The model under review builds one solid part; all positions refer to its coordinate system, in mm. A direction names the side the tool comes from. Coordinates: 2 decimals unless noted, no trailing zeros. Put each result on its own line as item: value.
from build123d import *

# Parameters (mm, degrees)
F1_DEPTH       = 6
F2_R           = 1
F3_D           = 2.8
F3_CBORE_D     = 6
F3_CBORE_DEPTH = 2.5
F4_R           = 5
F5_DEPTH       = 1.8
F7_D           = 2.8
F7_CBORE_D     = 6
F7_CBORE_DEPTH = 2.5
F8_SIZE        = 3
F10_DEPTH      = 0.4
F11_W          = 2
F11_H          = 59
F12_DEPTH      = 2
F13_SIZE       = 1.99999


# Not quite as in the source:
# - a fillet or chamfer is up to 0.001 mm smaller than in the source, because OpenCascade refuses the exact size


with BuildPart() as f1:
    # F0 (on Right) → F1 (new body)
    with BuildSketch(Plane.YZ):
        Polygon((40.0512183458, -60), (50, -60), (50, 60), (-50, 60), (-50, -60), (-40, -60), (-29.9487816542, -50), (30.0512183458, -50), align=None)
        with BuildLine():
            Line((2.1213203436, -9.1923881554), (32.9289321881, -40))
            Line((32.9289321881, -40), (-32.9289321881, -40))
            Line((-32.9289321881, -40), (-2.1213203436, -9.1923881554))
            ThreePointArc((-2.1213203436, -9.1923881554), (0, -8.313708499), (2.1213203436, -9.1923881554))
        make_face(mode=Mode.SUBTRACT)
        with BuildLine():
            Line((-9.1923881554, -2.1213203436), (-40, -32.9289321881))
            Line((-40, -32.9289321881), (-40, 32.9289321881))
            Line((-40, 32.9289321881), (-9.1923881554, 2.1213203436))
            ThreePointArc((-9.1923881554, 2.1213203436), (-8.313708499, 0), (-9.1923881554, -2.1213203436))
        make_face(mode=Mode.SUBTRACT)
        with BuildLine():
            Line((40, 32.9289321881), (40, -32.9289321881))
            Line((40, -32.9289321881), (9.1923881554, -2.1213203436))
            ThreePointArc((9.1923881554, -2.1213203436), (8.313708499, 0), (9.1923881554, 2.1213203436))
            Line((9.1923881554, 2.1213203436), (40, 32.9289321881))
        make_face(mode=Mode.SUBTRACT)
        with BuildLine():
            Line((-32.9289321881, 40), (32.9289321881, 40))
            Line((32.9289321881, 40), (2.1213203436, 9.1923881554))
            ThreePointArc((2.1213203436, 9.1923881554), (0, 8.313708499), (-2.1213203436, 9.1923881554))
            Line((-2.1213203436, 9.1923881554), (-32.9289321881, 40))
        make_face(mode=Mode.SUBTRACT)
    extrude(amount=F1_DEPTH)

    # F2
    f2_edges = [f1.edges().sort_by_distance(p)[0] for p in [
        (3, -32.928932, 40),
        (3, 32.928932, 40),
        (3, -40, 32.928932),
        (3, -40, -32.928932),
        (3, -32.928932, -40),
        (3, 40, 32.928932),
        (3, 40, -32.928932),
        (3, 32.928932, -40),
    ]]
    fillet(f2_edges, radius=F2_R)

    # F3 (through all)
    with Locations(Plane(origin=(0, 0, 0), x_dir=(0, 1, 0), z_dir=(-1, 0, 0))):
        with Locations((-40, -50), (40, -50)):
            CounterBoreHole(F3_D / 2, F3_CBORE_D / 2, F3_CBORE_DEPTH)

    # F4 (on face) → F5 (cut)
    with BuildSketch(Plane(origin=(0, 0, 0), x_dir=(0, -1, 0), z_dir=(-1, 0, 0))):
        Circle(F4_R)
    extrude(amount=-F5_DEPTH, mode=Mode.SUBTRACT)

    # F7 (through all)
    with Locations(Plane(origin=(0, 0, 0), x_dir=(0, -1, 0), z_dir=(-1, 0, 0))):
        with Locations((-5, -45), (5, -45)):
            CounterBoreHole(F7_D / 2, F7_CBORE_D / 2, F7_CBORE_DEPTH)

    # F8
    f8_edges = [f1.edges().sort_by_distance(p)[0] for p in [
        (3, -50, 60),
        (3, 50, 60),
        (0, -50, 0),
        (0, 50, 0),
        (0, 0, 60),
    ]]
    chamfer(f8_edges, length=F8_SIZE)

    # F9 (on face) → F10 (join)
    with BuildSketch(Plane(origin=(0, 0, 0), x_dir=(0, -1, 0), z_dir=(-1, 0, 0))):
        with BuildLine():
            Line((-47, 57), (-37, 57))
            ThreePointArc((-37, 57), (-54.0710678119, 64.0710678119), (-47, 47))
            Line((-47, 47), (-47, 57))
        make_face()
        with BuildLine():
            ThreePointArc((47, 47), (54.0710678119, 64.0710678119), (37, 57))
            Line((37, 57), (47, 57))
            Line((47, 57), (47, 47))
        make_face()
        with BuildLine():
            Line((-47, -60), (-47, -50))
            ThreePointArc((-47, -50), (-53.0480452096, -67.9637396456), (-37.3669885172, -57.3157701715))
            Line((-37.3669885172, -57.3157701715), (-40.0512183458, -60))
            Line((-40.0512183458, -60), (-47, -60))
        make_face()
        with BuildLine():
            ThreePointArc((37.3529996858, -57.3664880981), (53.0689735945, -67.9478021811), (47, -50))
            Line((47, -50), (47, -60))
            Line((47, -60), (40, -60))
            Line((40, -60), (37.3529996858, -57.3664880981))
        make_face()
    extrude(amount=-F10_DEPTH)

    # F11 (on face) → F12 (cut)
    with BuildSketch(Plane.XY.offset(60)):
        with Locations((5, -2.5)):
            Rectangle(F11_W, F11_H)
    extrude(amount=-F12_DEPTH, mode=Mode.SUBTRACT)

    # F13 (size 2 in the source; OpenCascade refuses exactly that, so slightly less here)
    f13_edges = [f1.edges().sort_by_distance(p)[0] for p in [
        (4, -2.5, 58),
        (5, 27, 58),
        (5, -32, 58),
    ]]
    chamfer(f13_edges, length=F13_SIZE)


solid = f1.part
Item 1: For line 1 (Y direction, x = 3.7, z = 50); line 2 (Z direction, x = 5.25, y = -5); line 3 (Z direction, x = 2.5, y = 20), list the stretches that pass through material, from the lowest coordinate up. Write a range as from..to.
Answers below:
line 1: -50..-41.4, -38.6..38.6, 41.4..50
line 2: -50..-46.4, -43.6..-40, -12.07..12.07, 40..58.75
line 3: -50..-40, -27.07..-12.93, 12.93..27.07, 40..59.5
Item 2: Mouldability with a two-part tool opening along Y and no side actions: class faces 4 (the flat face through (3, 0, -40)), 5 (the cylindrical face through (4.27, -5.18, -43.61)), 6 (the flat face through (4, -50, -1)), 7 (the flat face through (3, 45, -60)) as +Y half, -Y half, draft (parallel to the pull), parting line (faces both ways), or undercut.
Answers below:
face 4: undercut
face 5: undercut
face 6: -Y half
face 7: draft
Item 3: For pin 1 Ø1.8 at (y, z) = (6, -45) entering from -X; pin 2 Ø1.8 at (x, y) = (3, -4) entering from +Z; pin 3 Ø3 at (x, y) = (3.5, 24.5) entering from -Z, all flat-tipped, find the tip position at first contact; note any pin that passes through.
Answers below:
pin 1: x = 2.5
pin 2: z = 60
pin 3: z = -50
Item 4: Consider section A-A on y = -25. Count the separate pieces of the cut face and the enclosed holes in it, and give its area (3 significant figures).
Answers below:
separate pieces: 4
enclosed holes: 0
area: 343 mm^2
Item 5: For faces 1 (the flat face through (0, 13, -16)), 2 (the flat face through (4, -49, 58)), 3 (the flat face through (3, 40, 0)), list the 3-axis set-ups (+Z, -Z, +X, -X, +Y, -Y) from which the entire face can be reached by the end or side of a thin tool; tool diameter is ignored.
Answers below:
face 1: +Z, -Z, -X, +Y, -Y
face 2: +Z, +X, -Y
face 3: +X, -X
